Can you work these out from the drawing? Everything is in mm from the part's minimum corner. Coordinates: 2 decimals unless noted, no trailing zeros. Order: outer loops, then holes, each group sorted by start corner. A loop starts at its lowest first (then second) coordinate and runs counter-clockwise, first axis right, second up. Notation, with made-up numbers: (57.5, 42) -> (103.5, 42) arc R25 cw to (103.5, 62) -> close; hole circle Ø11 at (13, 53.5). An arc over 180 degrees is marked (long way). Write item = value, one per line. Start each with the question number.
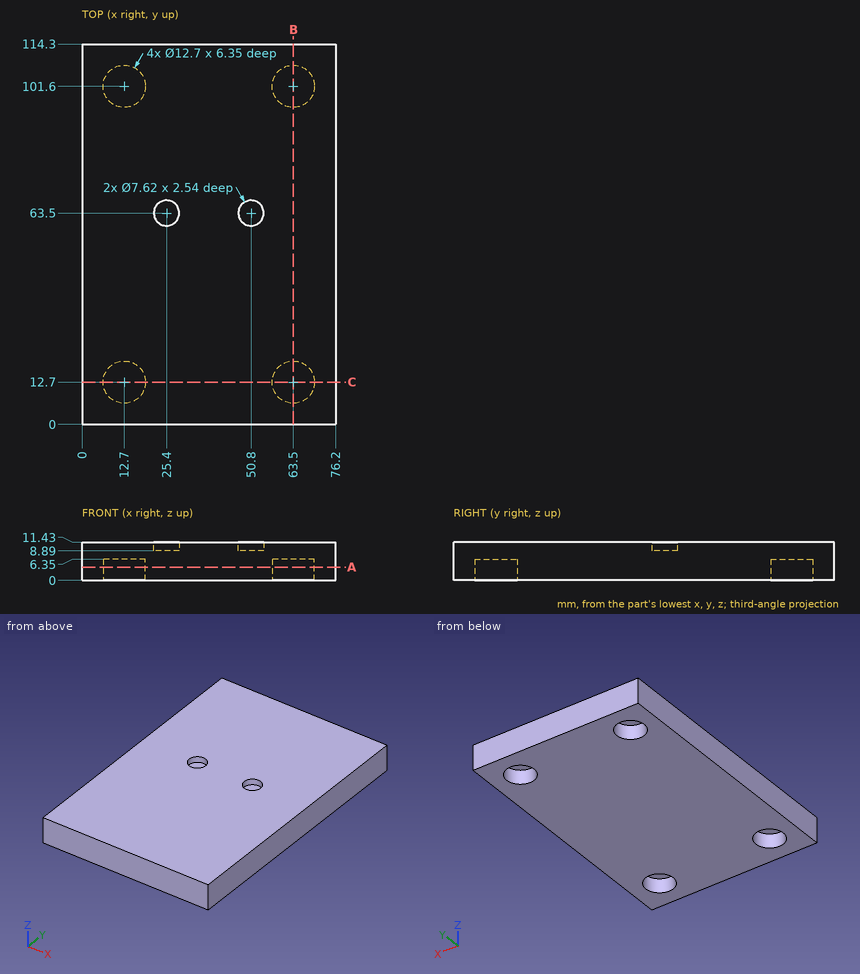
(1) Imagine slicing it at A-A (z = 4). Write out the boundary of the cut face in (x, y).
(2) For P1, Ø6.5, axis at x = 62, y = 16, coming from the -Z side; P2, Ø6.5, axis at x = 63, y = 103.5, coming from the -Z side, each with a flat end and sliding along its axis, tell me the tip position at first contact or that it passes through.
(3) If I drill on L1, parallel to Y at x = 63.5, z = 4.25; L2, parallel to X at y = 101.6, z = 3.75; L3, parallel to Y at x = 50.8, z = 9.55, over which ranges is the centre line in solid material (lowest first)? Write a range as from..to.
(4) Imagine slicing it at C-C (y = 12.7). Write out the boundary of the cut face in (x, z), plus the area to 3 significant figures.
(5) Imagine slicing it at B-B (x = 63.5). Write out the boundary of the cut face in (y, z), plus the area to 3 significant figures.
Result set:
q1.outline = (0, 0) -> (76.2, 0) -> (76.2, 114.3) -> (0, 114.3) -> close; hole circle Ø12.7 at (12.7, 12.7); hole circle Ø12.7 at (12.7, 101.6); hole circle Ø12.7 at (63.5, 12.7); hole circle Ø12.7 at (63.5, 101.6)
q2.P1 = 0
q2.P2 = 6.35
q3.L1 = 0..6.35, 19.05..95.25, 107.95..114.3
q3.L2 = 0..6.35, 19.05..57.15, 69.85..76.2
q3.L3 = 0..59.69, 67.31..114.3
q4.outline = (0, 0) -> (6.35, 0) -> (6.35, 6.35) -> (19.05, 6.35) -> (19.05, 0) -> (57.15, 0) -> (57.15, 6.35) -> (69.85, 6.35) -> (69.85, 0) -> (76.2, 0) -> (76.2, 11.43) -> (0, 11.43) -> close
q4.area = 710 mm2
q5.outline = (0, 0) -> (6.35, 0) -> (6.35, 6.35) -> (19.05, 6.35) -> (19.05, 0) -> (95.25, 0) -> (95.25, 6.35) -> (107.95, 6.35) -> (107.95, 0) -> (114.3, 0) -> (114.3, 11.43) -> (0, 11.43) -> close
q5.area = 1,150 mm2
